from build123d import *

# Parameters (mm, degrees)
SKETCH1_W           = 350
SKETCH1_H           = 50
BOSS_EXTRUDE1_DEPTH = 3
BOSS_EXTRUDE2_DEPTH = 350
SKETCH3_OUTSIDE_W   = 128.892
SKETCH3_OUTSIDE_H   = 422.892
SKETCH3_OUTSIDE_W_2 = 56
SKETCH3_OUTSIDE_H_2 = 350
SKETCH3_OUTSIDE_W_3 = 12.5
SKETCH3_OUTSIDE_H_3 = 3.5
SKETCH3_OUTSIDE_W_4 = 3.5
SKETCH3_OUTSIDE_H_4 = 12.5
CUT_EXTRUDE2_DEPTH  = 178.251234128


with BuildPart() as part:
    # Sketch1 → Boss-Extrude1 (new body)
    with BuildSketch(Plane(origin=(0, 0, 0), x_dir=(0, 1, 0), z_dir=(0, 0, 1))):
        Rectangle(SKETCH1_W, SKETCH1_H)
    extrude(amount=BOSS_EXTRUDE1_DEPTH)

    # Sketch2 → Boss-Extrude2 (add, through all)
    with BuildSketch(Plane.XZ.offset(175)):
        Polygon((-25, 3), (-25, 0), (-28, 0), align=None)
        Polygon((25, 3), (28, 0), (25, 0), align=None)
    extrude(amount=-BOSS_EXTRUDE2_DEPTH)

    # Sketch3 outside → Cut-Extrude2 (cut, through all)
    # profile 1 of 3: a face of its own
    with BuildSketch(Plane(origin=(0, 0, 0), x_dir=(1, 0, 0), z_dir=(0, 0, -1))):
        Rectangle(SKETCH3_OUTSIDE_W, SKETCH3_OUTSIDE_H)
        Rectangle(SKETCH3_OUTSIDE_W_2, SKETCH3_OUTSIDE_H_2, mode=Mode.SUBTRACT)
    # profile 2 of 3: a face of its own
    with BuildSketch(Plane(origin=(0, 0, 0), x_dir=(1, 0, 0), z_dir=(0, 0, -1))):
        with Locations((1.788055669, 5.25)):
            Rectangle(SKETCH3_OUTSIDE_W_3, SKETCH3_OUTSIDE_H_3)
    # profile 3 of 3: a face of its own
    with BuildSketch(Plane(origin=(0, 0, 0), x_dir=(1, 0, 0), z_dir=(0, 0, -1))):
        with Locations((-4.440759591, -64.557376571)):
            Rectangle(SKETCH3_OUTSIDE_W_4, SKETCH3_OUTSIDE_H_4)
    extrude(amount=-CUT_EXTRUDE2_DEPTH, mode=Mode.SUBTRACT)


solid = part.part
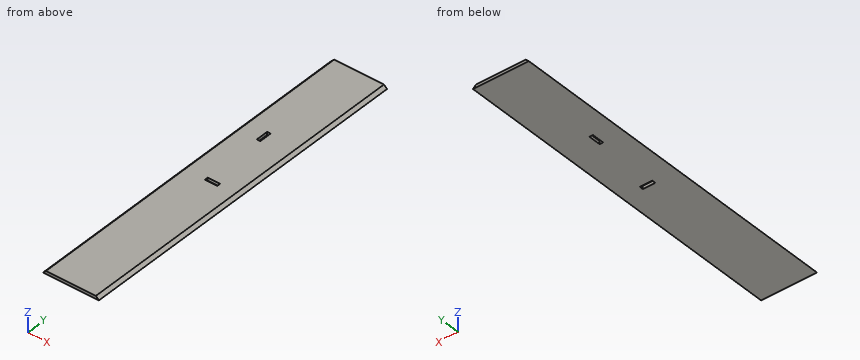
The model under review builds one solid part; all positions refer to its coordinate system, in mm. Give positions to 0.01 mm unless a question says otherwise; leave off trailing zeros. Write each loop counter-clockwise with the first axis right and the second up, starting at its lowest first coordinate (ties: lowest second). Pieces come first, ordered by that corner, then holes.
1. Add section B-B, the plane y = -48.5. Write out the cut boundary in (x, z), plus the area to 3 significant figures.
2. Wall thickness on L1, parallel to Y at x = -3, z = 0.25; L2, parallel to Y at x = -5.5, z = 1.6; L3, parallel to Y at x = 7.5, z = 1.9: over which ranges is each line inside the solid? List them lowest first.
3. For P1, Ø1.5, axis at y = -6, z = 2, coming from the +X side; P2, Ø0.9, axis at y = 64, z = 1.5, coming from the +X side; P3, Ø1, axis at y = -89, z = 1, coming from the +X side, all flat-tipped, find the tip position at first contact; note any pin that passes through.
4. Add section A-A, the plane z = 2.05. Write out the cut boundary in (x, y).
Worked answers:
1. outline: (-28, 0) - (28, 0) - (25, 3) - (-25, 3) - close
1. area: 159 mm2
2. L1: y = -175 to -7, -3.5 to 58.31, 70.81 to 175
2. L2: y = -175 to 58.31, 70.81 to 175
2. L3: y = -175 to -7, -3.5 to 175
3. P1: stops at x = 26.75
3. P2: stops at x = 26.95
3. P3: stops at x = 27.5
4. outline: (-25.95, -175) - (25.95, -175) - (25.95, 175) - (-25.95, 175) - close; hole (-6.19, 58.31) - (-2.69, 58.31) - (-2.69, 70.81) - (-6.19, 70.81) - close; hole (-4.46, -7) - (8.04, -7) - (8.04, -3.5) - (-4.46, -3.5) - close
